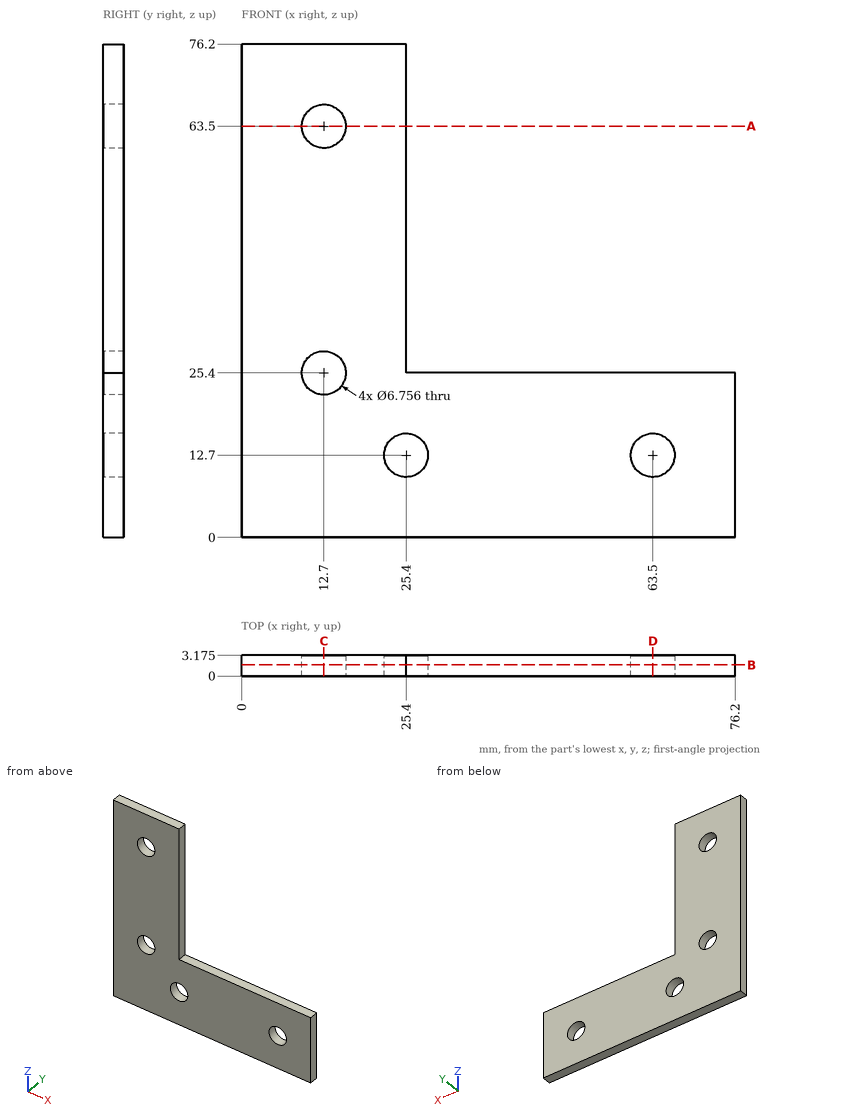
Verification items for this drawing (mm, ordinates from the low corner). Give positions to 0.01 mm unless a question says otherwise; leave off trailing zeros. Loops run counter-clockwise (first coordinate to the right, second up) from the corner with the lowest first, then second, coordinate; pieces in that order, holes last. Notation, with made-up numbers: M 65.25,58.25 L 88.25,58.25 A26 cw 88.25,92.25 Z; hole C 3.25,70 d10. An arc over 180 degrees is marked long. Return JSON: item names as keys, results as strings. Group by question number.
1. Cross-section at A-A on z = 63.5. Record the boundary of the cut face in (x, y) (1 decimal).
2. Thickness scan on L1, parallel to Z at x = 63.5, y = 2.7; L2, parallel to Z at x = 13.5, y = 1.15; L3, parallel to X at y = 3, z = 62. Record the ranges inside material, lowest first.
3. Cross-section at D-D on x = 63.5. Record the boundary of the cut face in (y, z) (1 decimal).
4. Cross-section at B-B on y = 1.7. Record the boundary of the cut face in (x, z).
5. Go/stop test with a flat-tipped pin: pin 1 (1.6 mm diameter, centred on y = 1.5, z = 53.5, fed in from +X). Record where the tip stops, or that it passes through.
6. Cross-section at C-C on x = 12.7. Record the boundary of the cut face in (y, z) (1 decimal), plus the area to 3 significant figures.
Return value:
{
 "1": {"outline": "M 0,0 L 9.3,0 L 9.3,3.2 L 0,3.2 Z; M 16.1,0 L 25.4,0 L 25.4,3.2 L 16.1,3.2 Z"},
 "2": {"L1": "0 to 9.32, 16.08 to 25.4", "L2": "0 to 22.12, 28.68 to 60.22, 66.78 to 76.2", "L3": "0 to 9.67, 15.73 to 25.4"},
 "3": {"outline": "M 0,0 L 3.2,0 L 3.2,9.3 L 0,9.3 Z; M 0,16.1 L 3.2,16.1 L 3.2,25.4 L 0,25.4 Z"},
 "4": {"outline": "M 0,0 L 76.2,0 L 76.2,25.4 L 25.4,25.4 L 25.4,76.2 L 0,76.2 Z; hole C 12.7,25.4 d6.76; hole C 12.7,63.5 d6.76; hole C 25.4,12.7 d6.76; hole C 63.5,12.7 d6.76"},
 "5": {"pin 1": "x = 25.4"},
 "6": {"outline": "M 0,0 L 3.2,0 L 3.2,22 L 0,22 Z; M 0,28.8 L 3.2,28.8 L 3.2,60.1 L 0,60.1 Z; M 0,66.9 L 3.2,66.9 L 3.2,76.2 L 0,76.2 Z", "area": "199 mm^2"}
}
